The figure shows three views and two pictorial views of one solid part (mm, origin at its lowest corner). Answer the questions. A direction names the side the tool comes from. Coordinates: 2 decimals unless noted, no trailing zeros. Write each loop counter-clockwise with the first axis right and the second up, starting at its lowest first coordinate (ties: lowest second). Pieces come first, ordered by that corner, then holes. Notation, with made-up numbers: M 20.25,48 L 35.25,48 A19 ccw 35.25,70 Z; hole C 33,-33.5 d6. An arc over 180 degrees is marked long. Write item = value, one per line.
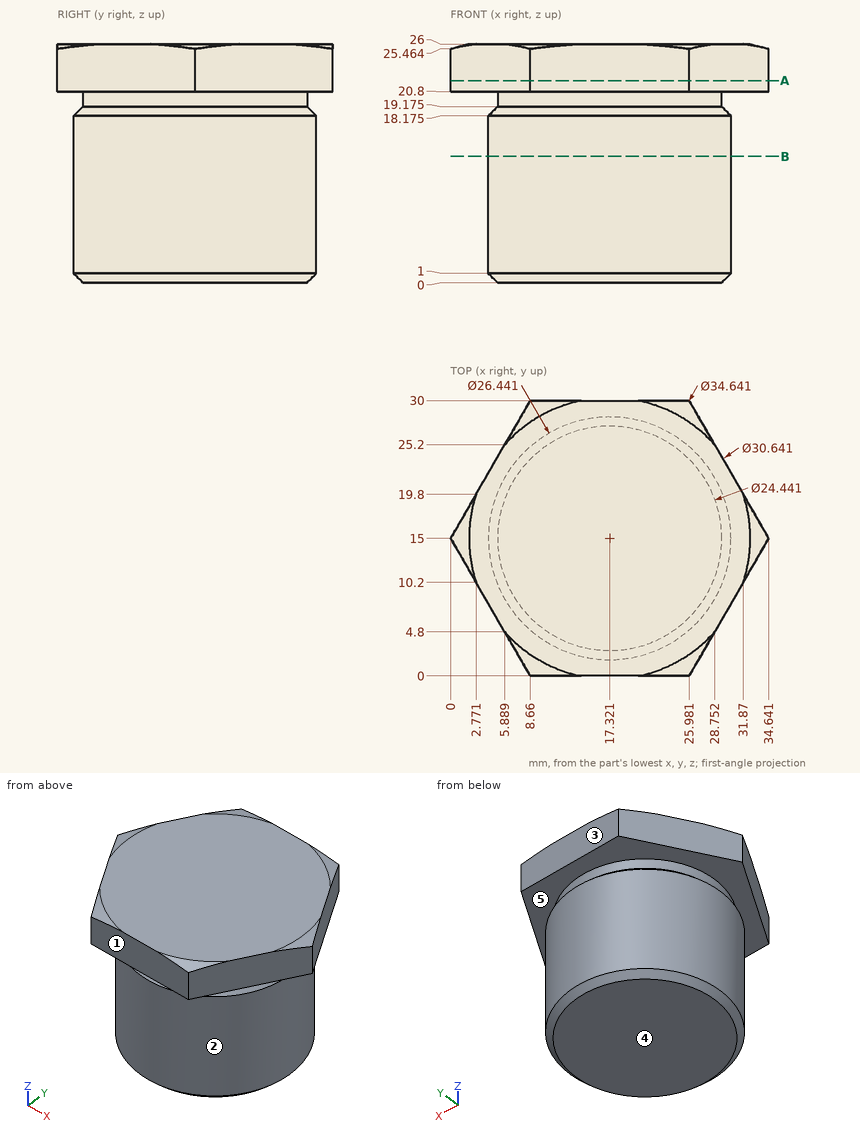
Item 1: Find section B-B (z = 13.75). Determine the outline of the cut face in (x, y).
Worked answers:
outline = C 17.32,15 d26.44
Item 2: Flat-ended cylindrical pins translate along their axes: pin 1 (2 mm diameter, centred on y = 18, z = 13, fed in from +X); pin 2 (8 mm diameter, centred on y = 7.5, z = 21, fed in from +X); pin 3 (8 mm diameter, centred on y = 26, z = 7, fed in from -X) (1 decimal). Find the tip coordinate at first contact, or state that the pin passes through.
Worked answers:
pin_1 = 30.39
pin_2 = 32.62
pin_3 = 6.1
Item 3: Find section A-A (z = 22). Determine the outline of the cut face in (x, y).
Worked answers:
outline = M 0,15 L 8.66,0 L 25.98,0 L 34.64,15 L 25.98,30 L 8.66,30 Z
Item 4: Which of the six approach directions +Z, -Z, +X, -X, +Y, -Y give full straight-line access (tool end or side, diameter ignored) to the marked faces 1 and 2?
Worked answers:
face_1 = +Z, -Z, +X, -X, -Y
face_2 = -Z
Item 5: For a pull along Z with two mould halves and no side action, classify the marked faces 3, 4 and 5 as released by +Z, released by -Z, zero draft, split by the parting line, or undercut.
Worked answers:
face_3 = zero draft
face_4 = released by -Z
face_5 = undercut
Item 6: Consider line 1 along Z through (x, y) = (28, 25); line 2 along X through (y, z) = (21, 2.5); line 3 along Y through (x, z) = (16.5, 14) (1 decimal). Determine where each line is inside the solid, lowest interval first. Write a range as from..to.
Worked answers:
line_1 = 20.8..26
line_2 = 5.54..29.1
line_3 = 1.8..28.2
